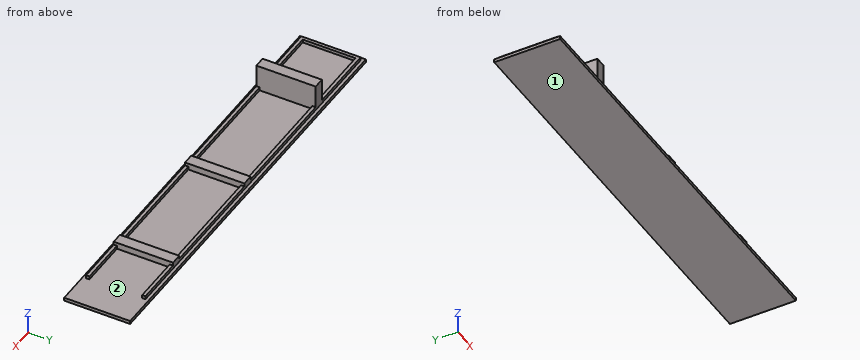
Autodesk Fusion 360 part; units mm, degrees
sketch "Sketch1" plane through (0, 0, 0) normal (0, 0, 1) x (1, 0, 0)
  line L0 (0, 0) -> (190, 0)
  line L1 (190, 0) -> (190, 30)
  line L2 (190, 30) -> (0, 30)
  line L3 (0, 30) -> (0, 0)
  dimension "d1" = 190
  dimension "d2" = 30
extrude "Extrude1" add sketch "Sketch1" along normal blind 1.5
sketch "Sketch2" plane through (0, 0, 1.5) normal (0, 0, 1) x (-1, 0, 0)
  line L0 (0, -30) -> (0, 0)
  line L1 (0, 0) -> (-190, 0)
  line L2 (-190, 0) -> (-190, -30)
  line L3 (-190, -30) -> (0, -30)
  line L4 (-1.5, -1.5) -> (-188.5, -1.5)
  line L5 (-188.5, -1.5) -> (-188.5, -28.5)
  line L6 (-188.5, -28.5) -> (-1.5, -28.5)
  line L7 (-1.5, -28.5) -> (-1.5, -1.5)
  line L8 (-32.75, -28.5) -> (-37.75, -28.5)
  line L9 (-37.75, -28.5) -> (-37.75, -1.5)
  line L10 (-37.75, -1.5) -> (-32.75, -1.5)
  line L11 (-32.75, -1.5) -> (-32.75, -28.5)
  line L12 (-188.5, -28.5) -> (-157.25, -28.5)
  line L13 (-90.25, -28.5) -> (-95.25, -28.5)
  line L14 (-90.25, -1.5) -> (-90.25, -28.5)
  line L15 (-95.25, -28.5) -> (-95.25, -1.5)
  line L16 (-95.25, -1.5) -> (-90.25, -1.5)
  line L17 (-147.75, -28.5) -> (-152.75, -28.5)
  line L18 (-147.75, -1.5) -> (-147.75, -28.5)
  line L19 (-152.75, -28.5) -> (-152.75, -1.5)
  line L20 (-152.75, -1.5) -> (-147.75, -1.5)
  dimension "d5" = -1.5
  dimension "d6" = 5
  dimension "d7" = 31.25
  dimension "d8" = 31.25
  dimension "d11" = -115
  dimension "d12" = 0
extrude "Extrude2" add sketch "Sketch2" along normal blind 12 contours L4 L6 L8 L9 L10 L11
extrude "Extrude3" add sketch "Sketch2" along normal blind 3 contours L4 L6 L13 L14 L15 L16 | L4 L6 L17 L18 L19 L20
extrude "Extrude4" add sketch "Sketch2" along normal blind 1.5 contours L4 L6 L7 L11
sketch "Sketch3" plane through (0, 0, 3) normal (0, 0, 1) x (-1, 0, 0)
  line L0 (-32.75, -1.5) -> (-32.75, -28.5)
  line L1 (-32.75, -28.5) -> (-1.5, -28.5)
  line L2 (-1.5, -28.5) -> (-1.5, -1.5)
  line L3 (-1.5, -1.5) -> (-32.75, -1.5)
  line L4 (-3, -3) -> (-31.25, -3)
  line L5 (-31.25, -27) -> (-3, -27)
  line L6 (-3, -27) -> (-3, -3)
  line L7 (-31.25, -3) -> (-32.75, -3)
  line L8 (-31.25, -27) -> (-32.75, -27)
extrude "Extrude5" cut sketch "Sketch3" against normal blind 1.5 contours L0 L4 L5 L6 L7 L8
sketch "Sketch4" plane through (0, 0, 1.5) normal (0, 0, 1) x (-1, 0, 0)
  line L0 (0, -30) -> (0, 0)
  line L1 (0, 0) -> (-190, 0)
  line L2 (-190, 0) -> (-190, -30)
  line L3 (-190, -30) -> (0, -30)
  line L4 (-37.75, -1.5) -> (-1.5, -1.5)
  line L5 (-1.5, -1.5) -> (-1.5, -28.5)
  line L6 (-1.5, -28.5) -> (-37.75, -28.5)
  line L7 (-37.75, -28.5) -> (-37.75, -1.5)
  line L8 (-95.25, -1.5) -> (-90.25, -1.5)
  line L9 (-90.25, -1.5) -> (-90.25, -28.5)
  line L10 (-90.25, -28.5) -> (-95.25, -28.5)
  line L11 (-95.25, -28.5) -> (-95.25, -1.5)
  line L12 (-152.75, -1.5) -> (-147.75, -1.5)
  line L13 (-147.75, -1.5) -> (-147.75, -28.5)
  line L14 (-147.75, -28.5) -> (-152.75, -28.5)
  line L15 (-152.75, -28.5) -> (-152.75, -1.5)
  line L16 (-190, -28.5) -> (-37.75, -28.5)
  line L17 (-37.75, -28.5) -> (-37.75, -27)
  line L18 (-37.75, -27) -> (-190, -27)
  line L19 (-190, -27) -> (-190, -28.5)
  line L20 (-190, -1.5) -> (-37.75, -1.5)
  line L21 (-37.75, -1.5) -> (-37.75, -3)
  line L22 (-37.75, -3) -> (-190, -3)
  line L23 (-190, -3) -> (-190, -1.5)
  line L24 (0, 0) -> (-190, 0)
  line L25 (-190, -30) -> (0, -30)
  line L26 (-95.25, -28.5) -> (-95.25, -1.5)
  line L27 (-37.75, -28.5) -> (-37.75, -1.5)
  line L28 (-175, -28.5) -> (-175, -27)
  line L29 (-175, -3) -> (-175, -1.5)
  line L30 (-190, 0) -> (-190, -30)
  dimension "d22" = 1.5
  dimension "d23" = 1.5
  dimension "d24" = 1.5
  dimension "d25" = 1.5
  dimension "d26" = 15
  dimension "d27" = 15
extrude "Extrude6" add sketch "Sketch4" along normal blind 1.5 contours L15 L16 L18 L28 | L15 L20 L22 L29 | L11 L13 L16 L18 L26 | L11 L13 L20 L22 L26 | L7 L9 L16 L17 L18 L27 | L7 L9 L20 L21 L22 L27
component "Lid" placed x (1, 0, 0) y (0, 1, 0) z (0, 0, 1) at (0, 0, 0)
Verification items for the finished model (mm, model axes). Face numbers are marked on the shaded views. Coordinates: 2 decimals unless noted, no trailing zeros. Order: outer loops, then holes, each group sorted by start corner. A loop starts at its lowest first (then second) coordinate and runs counter-clockwise, first axis right, second up. Notation, with made-up numbers: (76, -9.5) - (114, -9.5) arc R17 cw to (114, -2.5) - close; hole circle Ø3 at (28, -7). An arc over 180 degrees is marked (long way). Return JSON: item names as keys, results as strings.
(1) Mould release check, pull along Y, two halves, no side actions. Record for the marked faces 1 and 2: pulls with the +Y half, pulls with the -Y half, needs draft (parallel to the pull), parting line crosses it, or undercut.
Filled sheet:
{"face 1": "needs draft", "face 2": "undercut"}
(2) Section check A-A, the plane x = 35. Record the cut outline in (y, z), and give its area (3 significant figures).
Filled sheet:
{"outline": "(0, 0) - (30, 0) - (30, 1.5) - (28.5, 1.5) - (28.5, 13.5) - (1.5, 13.5) - (1.5, 1.5) - (0, 1.5) - close", "area": "369 mm^2"}
(3) Section check D-D, the plane x = 108. Record the cut outline in (y, z).
Filled sheet:
{"outline": "(0, 0) - (30, 0) - (30, 1.5) - (28.5, 1.5) - (28.5, 3) - (27, 3) - (27, 1.5) - (3, 1.5) - (3, 3) - (1.5, 3) - (1.5, 1.5) - (0, 1.5) - close"}
(4) Go/stop test with flat-tipped pins: pin 1 (7 mm diameter, centred on x = 120, y = 10.5, fed in from +Z); pin 2 (1.6 mm diameter, centred on x = 159, z = 2.5, fed in from -Y); pin 3 (1.5 mm diameter, centred on y = 20, z = 3, fed in from +X); pin 4 (2 mm diameter, centred on x = 28, z = 5, fed in from +Y). Record where each tip stops, or that it passes through.
Filled sheet:
{"pin 1": "stops at z = 1.5", "pin 2": "stops at y = 1.5", "pin 3": "stops at x = 152.75", "pin 4": "passes through"}
(5) Thickness scan on line 1 along X through (y, z) = (12.5, 1.75); line 2 along Y through (x, z) = (128.5, 2.75); line 3 along Z through (x, y) = (67, 23.25). Record the ranges inside material, lowest first.
Filled sheet:
{"line 1": "x = 1.5 to 3, 32.75 to 37.75, 90.25 to 95.25, 147.75 to 152.75", "line 2": "y = 1.5 to 3, 27 to 28.5", "line 3": "z = 0 to 1.5"}
(6) Section check C-C, the plane z = 7. Record the cut outline in (x, y).
Filled sheet:
{"outline": "(32.75, 1.5) - (37.75, 1.5) - (37.75, 28.5) - (32.75, 28.5) - close"}
(7) Section check B-B, the plane y = 11.25. Record the cut outline in (x, z), and give its area (3 significant figures).
Filled sheet:
{"outline": "(0, 0) - (190, 0) - (190, 1.5) - (152.75, 1.5) - (152.75, 4.5) - (147.75, 4.5) - (147.75, 1.5) - (95.25, 1.5) - (95.25, 4.5) - (90.25, 4.5) - (90.25, 1.5) - (37.75, 1.5) - (37.75, 13.5) - (32.75, 13.5) - (32.75, 1.5) - (3, 1.5) - (3, 3) - (1.5, 3) - (1.5, 1.5) - (0, 1.5) - close", "area": "377 mm^2"}
